The model under review builds one solid part; all positions refer to its coordinate system, in mm. A direction names the side the tool comes from. Coordinates: 2 decimals unless noted, no trailing zeros. Loops run counter-clockwise (first coordinate to the right, second up) from the corner with the lowest first, then second, coordinate; pieces in that order, holes last. Notation, with made-up numbers: M 48,35 L 66,35 A32 cw 66,73 Z; hole C -28,-19.5 d9. An arc over 180 degrees is marked long. Use one line per item in the form item = value.
Autodesk Inventor part; units mm, degrees
ref_plane "YZ Plane" through (0, 0, 0) normal (1, 0, 0) x (0, 1, 0)
ref_plane "XZ Plane" through (0, 0, 0) normal (0, 1, 0) x (-1, 0, 0)
ref_plane "XY Plane" through (0, 0, 0) normal (0, 0, 1) x (1, 0, 0)
sketch "Sketch1" plane through (0, 0, 0) normal (1, 0, 0) x (0, 1, 0)
  line L0 (0, 4.4) -> (0, -4.4)
  line L1 (0, -4.4) -> (-0.9, -4.4)
  line L2 (-0.9, -4.4) -> (-1.9, -3.4)
  line L3 (-1.9, -3.4) -> (-1.9, -3.4)
  line L4 (-1.9, -3.4) -> (-25, -3.4)
  line L5 (-25, -3.4) -> (-25, 3.4)
  line L6 (-25, 3.4) -> (-1.9, 3.4)
  line L7 (-1.9, 3.4) -> (-1.9, 3.4)
  line L8 (-1.9, 3.4) -> (-0.9, 4.4)
  line L9 (-0.9, 4.4) -> (0, 4.4)
  line L10 (0, 0) -> (-25, 0) construction
  line L11 (-24, 3.4) -> (-24, -3.4)
  line L12 (-12, 3.4) -> (-12, 0.75)
  line L13 (-12, 0.75) -> (-19, 0.75)
  line L14 (-19, 0.75) -> (-19, 2.6)
  line L15 (-19, 2.6) -> (-17, 2.6)
  line L16 (-17, 2.6) -> (-17, 3.4)
  line L17 (-12, -3.4) -> (-12, -0.75)
  line L18 (-12, -0.75) -> (-19, -0.75)
  line L19 (-19, -0.75) -> (-19, -2.6)
  line L20 (-19, -2.6) -> (-17, -2.6)
  line L21 (-17, -2.6) -> (-17, -3.4)
  dimension "d0" = 8.8
  dimension "d1" = 1.9
  dimension "d2" = 135
  dimension "d5" = 0.9
  dimension "d6" = 25
  dimension "d7" = 6.8
  dimension "d9" = 14
  dimension "d10" = 1
  dimension "d11" = 0.8
  dimension "d13" = 5
  dimension "d16" = 10
  dimension "d24" = 1.5
extrude "Extrusion1" add sketch "Sketch1" along normal mid plane 3.9
revolve "Revolution1" cut sketch "Sketch1" angle 360 about axis through (0, -24, 3.4) along (0, 0, -1) contours L12 L13 L14 L15 L16 L6 | L4 L21 L20 L19 L18 L17
fillet "Fillet1" radius 3 4 edges at (0, -12, 0.75) (0, -12, -0.75) (0, -25, -3.4) (0, -25, 3.4)
fillet "Fillet2" radius 0.3 4 edges at (0, -19, 2.6) (0, -19, 0.75) (0, -19, -0.75) (0, -19, -2.6)
sketch "Sketch2" plane through (1.95, 0, 0) normal (1, 0, 0) x (0, 0, -1)
  line L0 (-2.4, -1.9) -> (-2.4, -9.7595)
  line L1 (-2.4, -9.7595) -> (0, -12.1595)
  line L2 (0, -12.1595) -> (2.4, -9.7595)
  line L3 (2.4, -9.7595) -> (2.4, -1.9)
  line L4 (2.4, -1.9) -> (-2.4, -1.9)
  line L5 (-3.4, -1.9) -> (-3.4, -22)
  line L6 (0, 0) -> (0, -12.1595) construction
  line L7 (4.4, 0) -> (-4.4, 0)
  point P0 (-3.4, -12.1595)
  dimension "d19" = 1
  dimension "d20" = 135
extrude "Extrusion2" cut sketch "Sketch2" against normal through all
fillet "Fillet3" radius 0.5 5 edges at (0, -9.7595, 2.4) (0, -12.1595, 0) (0, -9.7595, -2.4) (0, -1.9, 2.4) (0, -1.9, -2.4)
properties part number "FS-04-SLBV1"
1. Add section C-C (y = -11). State the section outline as (x, z) points.
Response values:
outline = M -1.95,-3.4 L 1.95,-3.4 L 1.95,-1.16 L -1.95,-1.16 Z; M -1.95,1.16 L 1.95,1.16 L 1.95,3.4 L -1.95,3.4 Z
2. Insertion check: P1, Ø1, axis at x = 0, y = -13.5, coming from the +Z side; P2, Ø1.2, axis at x = 0, y = -6.5, coming from the +Z side; P3, Ø0.6, axis at x = 0.5, y = -17.5, coming from the -Z side. Each pin has a flat end and moves straight along its axis. Give the tip position at first contact, or say it passes through.
Response values:
P1 = 1.5
P2 = 3.4
P3 = -3.4
3. Add section B-B (z = -1.5). State the section outline as (x, y) points.
Response values:
outline = M -1.95,-24.79 L 1.95,-24.79 L 1.95,-19.4 A5 ccw -1.95,-19.4 Z; M -1.95,-13.17 A11 cw 1.95,-13.17 L 1.95,-10.66 L -1.95,-10.66 Z; M -1.95,-1.9 L 1.95,-1.9 L 1.95,0 L -1.95,0 Z
4. Wall thickness on line 1 along Z through (x, y) = (-1.6, -5.25); line 2 along Y through (x, z) = (1.7, -2.25); line 3 along Y through (x, z) = (0.8, -1.25): over which ranges is each line inside the solid? List them lowest first. Write a range as from..to.
Response values:
line_1 = -3.4..-2.4, 2.4..3.4
line_2 = -24.36..-19.3, -12.51..-9.91, -2.04..0
line_3 = -24.88..-19.06, -13.35..-10.91, -1.9..0
5. Add section A-A (y = -4). State the section outline as (x, z) points, then the cut area to 3 significant figures.
Response values:
outline = M -1.95,-3.4 L 1.95,-3.4 L 1.95,-2.4 L -1.95,-2.4 Z; M -1.95,2.4 L 1.95,2.4 L 1.95,3.4 L -1.95,3.4 Z
area = 7.80 mm^2
6. Machinability: for faces 4 (the face through (0, -20, 3.4)), 5 (the face through (0, -7, -3.4)), 6 (the face through (0, -6, 2.4)), 7 (the face through (0, -19, 2)), which of the approach directions +Z, -Z, +X, -X, +Y, -Y give a long, thin tool a straight path to every point of the face, cutting with its end or side? Answer none if there is none.
Response values:
face_4 = +Z, +X, -X, -Y
face_5 = -Z, +X, -X, -Y
face_6 = +X, -X
face_7 = none
7. The part is to be moulded in two halves that separate along Y. For faces 1 (the face through (0, -17, 0.75)), 2 (the face through (0, -7, 3.4)), 3 (the face through (-0.03, -24.1, -2.54)), say which applies: pulls with the +Y half, pulls with the -Y half, needs draft (parallel to the pull), parting line crosses it, or undercut.
Response values:
face_1 = undercut
face_2 = needs draft
face_3 = pulls with the -Y half
